Input: part model. Units: mm. Frame: model coordinates. Face numbers are marked on the shaded views. A direction names the side the tool comes from. Give positions to 0.01 mm unless a question says otherwise; leave off trailing zeros. Loops run counter-clockwise (first coordinate to the right, second up) from the corner with the lowest first, then second, coordinate; pieces in that order, holes last. Notation, with made-up numbers: (62.25, 65) -> (121.25, 65) arc R19 cw to (121.25, 80) -> close; hole circle Ø3 at (-32, 30.25). An arc over 180 degrees is marked (long way). Answer in a Markdown table with one row per item. Add a question column.
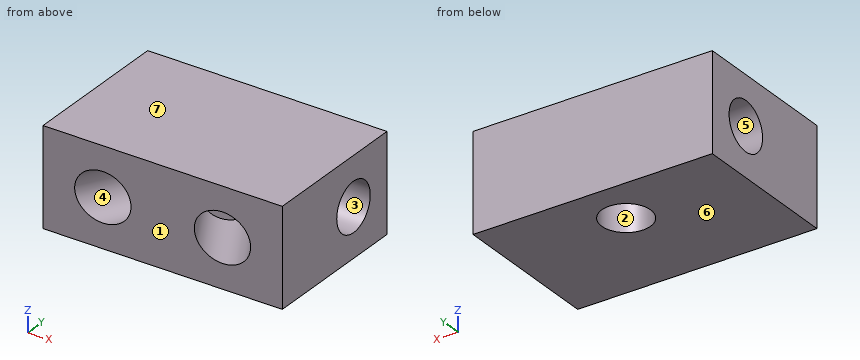
```python
from build123d import *

# Parameters (mm, degrees)
SKETCH3_W                      = 31.148374891
SKETCH3_H                      = 19.837641971
BOSS_EXTRUDE1_DEPTH            = 6.35
SKETCH4_R                      = 3.175
CUT_EXTRUDE1_DEPTH             = 9.525
SKETCH5_R                      = 3.175
CUT_EXTRUDE5_DEPTH             = 9.525
CUT_EXTRUDE5_DIRECTION_2_REACH = 33.299
SKETCH6_R                      = 3.175
CUT_EXTRUDE6_DEPTH             = 9.525


with BuildPart() as part:
    # Sketch3 → Boss-Extrude1 (new, symmetric)
    with BuildSketch(Plane.XY):
        with Locations((15.574187446, -9.918820986)):
            Rectangle(SKETCH3_W, SKETCH3_H)
    extrude(amount=BOSS_EXTRUDE1_DEPTH, both=True)

    # Sketch4 → Cut-Extrude1 (cut)
    with BuildSketch(Plane.ZY):
        with Locations(Location((0, -6.35, 0), (0, 0, 270))):
            Circle(SKETCH4_R)
    cut_extrude1 = extrude(amount=-CUT_EXTRUDE1_DEPTH, mode=Mode.SUBTRACT)

    # Sketch5 → Cut-Extrude5 (cut)
    with BuildSketch(Plane(origin=(7.787093723, -19.837641971, 0), x_dir=(-0.8660254037844382, 0.500000000000001, 0), z_dir=(-0.500000000000001, -0.8660254037844382, 0))):
        with Locations(Location((0, 0, 0), (0, 0, 180))):
            Circle(SKETCH5_R)
    cut_extrude5 = extrude(amount=-CUT_EXTRUDE5_DEPTH, mode=Mode.SUBTRACT)

    # Sketch5 → Cut-Extrude5 direction 2 (cut, up to next)
    with BuildSketch(Plane(origin=(7.787093723, -19.837641971, 0), x_dir=(-0.8660254037844382, 0.500000000000001, 0), z_dir=(-0.500000000000001, -0.8660254037844382, 0)), mode=Mode.PRIVATE) as cut_extrude5_direction_2_sk1:
        with Locations(Location((0, 0, 0), (0, 0, 180))):
            Circle(SKETCH5_R)
    cut_extrude5_direction_2_tool1 = extrude(cut_extrude5_direction_2_sk1.sketch, amount=CUT_EXTRUDE5_DIRECTION_2_REACH, mode=Mode.PRIVATE) & part.part
    cut_extrude5_direction_2 = cut_extrude5_direction_2_tool1.solids().sort_by_distance((7.787094, -19.837642, 0))[0]
    add(cut_extrude5_direction_2, mode=Mode.SUBTRACT)

    # Sketch6 → Cut-Extrude6 (cut)
    with BuildSketch(Plane(origin=(0, 0, -6.35), x_dir=(-1, 0, 0), z_dir=(0, 0, -1))):
        with Locations((-15.574187445, -6.35)):
            Circle(SKETCH6_R)
    extrude(amount=-CUT_EXTRUDE6_DEPTH, mode=Mode.SUBTRACT)

    # Mirror1: Cut-Extrude1, Cut-Extrude5, Cut-Extrude5 direction 2 across plane
    add(cut_extrude1.mirror(Plane.ZY.offset(-15.574187445)), mode=Mode.SUBTRACT)
    add(cut_extrude5.mirror(Plane.ZY.offset(-15.574187445)), mode=Mode.SUBTRACT)
    add(cut_extrude5_direction_2.mirror(Plane.ZY.offset(-15.574187445)), mode=Mode.SUBTRACT)


solid = part.part
```
1) Material intervals for line 1 along Z through (x, y) = (28, -6.35) (3 decimals); line 2 along Y through (x, z) = (15, 1); line 3 along Y through (x, z) = (13, -1), sorted ascending.
2) Section B-B on y = -6.35. Output: boundary loops of the cut face in (x, z) (3 decimals), and give its area (3 significant figures).
3) Reachability of the marked faces 1, 2 and 3 from +Z, -Z, +X, -X, +Y, -Y: full face, straight path, thin tool, end or side. Return the list, or none.
4) Pull-direction query (Z, two-part tool) for the marked faces 4, 5, 6 and 7; classes: +Z half, -Z half, draft (parallel to the pull), parting line (faces both ways), or undercut.
5) Section D-D on y = -17. State how many separate pieces and enclosed holes the cut face has, and give its area (3 significant figures).
6) Pin query (flat end, axial travel): pin 1 (1.9 mm diameter, centred on y = -6, z = 0, fed in from -X) (3 decimals); pin 2 (4 mm diameter, centred on y = -6.35, z = 0, fed in from +X). Return the tip coordinate at first contact, or that it passes through.
7) Section C-C on z = 0. Output: boundary loops of the cut face in (x, y) (3 decimals), and give its area (3 significant figures).
Working result:
| question | item | result |
|---|---|---|
| 1 | line 1 | z = -6.35 to -3.175, 3.175 to 6.35 |
| 1 | line 2 | y = -19.84 to -13.37, -13 to -9.47, -3.23 to 0 |
| 1 | line 3 | y = -19.84 to -16.84, -11.85 to -8.21, -4.49 to 0 |
| 2 | outline | (0, -6.35) -> (12.399, -6.35) -> (12.399, 3.175) -> (18.749, 3.175) -> (18.749, -6.35) -> (31.148, -6.35) -> (31.148, -3.175) -> (21.623, -3.175) -> (21.623, 3.175) -> (31.148, 3.175) -> (31.148, 6.35) -> (0, 6.35) -> (0, 3.175) -> (9.525, 3.175) -> (9.525, -3.175) -> (0, -3.175) -> close |
| 2 | area | 214 mm2 |
| 3 | face 1 | +Z, -Z, +X, -X, -Y |
| 3 | face 2 | -Z |
| 3 | face 3 | +X |
| 4 | face 4 | undercut |
| 4 | face 5 | undercut |
| 4 | face 6 | -Z half |
| 4 | face 7 | +Z half |
| 5 | separate pieces | 1 |
| 5 | enclosed holes | 2 |
| 5 | area | 322 mm2 |
| 6 | pin 1 | stops at x = 9.525 |
| 6 | pin 2 | stops at x = 21.62 |
| 7 | outline | (0, -19.838) -> (4.121, -19.838) -> (9.8, -10.001) -> (15.299, -13.176) -> (11.453, -19.838) -> (19.695, -19.838) -> (15.849, -13.176) -> (21.348, -10.001) -> (27.027, -19.838) -> (31.148, -19.838) -> (31.148, -9.525) -> (21.623, -9.525) -> (21.623, -3.175) -> (31.148, -3.175) -> (31.148, 0) -> (0, 0) -> (0, -3.175) -> (9.525, -3.175) -> (9.525, -9.525) -> (0, -9.525) -> close; hole circle Ø6.35 at (15.574, -6.35) |
| 7 | area | 344 mm2 |
